Could you check a few things on this model? Use its own coordinates, in mm. Coordinates: 2 decimals unless noted, no trailing zeros. Loops run counter-clockwise (first coordinate to the right, second up) from the corner with the lowest first, then second, coordinate; pieces in that order, holes last. Notation, with made-up numbers: (-2, 22) -> (20, 22) arc R29 cw to (20, 55) -> close; hole circle Ø4 at (50.25, -5). An arc over 180 degrees is marked (long way). One line per question, with ' | ' between items.
Autodesk Inventor part; units mm, degrees
ref_plane "YZ Plane" through (0, 0, 0) normal (1, 0, 0) x (0, 1, 0)
ref_plane "XZ Plane" through (0, 0, 0) normal (0, 1, 0) x (-1, 0, 0)
ref_plane "XY Plane" through (0, 0, 0) normal (0, 0, 1) x (1, 0, 0)
sketch "Sketch2" plane through (0, 0, 0) normal (0, 0, 1) x (1, 0, 0)
  line L0 (0, 0) -> (200, 0)
  line L1 (200, 0) -> (200, 100)
  line L2 (200, 100) -> (0, 100)
  line L3 (0, 100) -> (0, 0)
  line L4 (0, 5) -> (200, 5) construction
  line L5 (0, 95) -> (200, 95) construction
  circle A0 centre (12.5, 95) radius 2.25
  circle A1 centre (12.5, 5) radius 2.25
  circle A2 centre (187.5, 95) radius 2.25
  circle A3 centre (187.5, 5) radius 2.25
  point P0 (23, 5)
  point P1 (23, 95)
  point P2 (53, 5)
  point P3 (53, 95)
  point P4 (85, 95)
  point P5 (85, 5)
  point P6 (115, 95)
  point P7 (115, 5)
  point P8 (147, 95)
  point P9 (147, 5)
  point P10 (177, 95)
  point P11 (177, 5)
  dimension "d18" = 90
  dimension "d0" = 200
  dimension "d1" = 100
  dimension "d2" = 30
  dimension "d3" = 32
  dimension "d4" = 30
  dimension "d5" = 32
  dimension "d6" = 30
  dimension "d13" = 10.5
  dimension "d15" = 10.5
  dimension "d16" = 12.5
  dimension "d17" = 175
  dimension "d21" = 4.5
  dimension "d22" = 4.5
  dimension "d23" = 4.5
  dimension "d24" = 4.5
extrude "Extrusion2" add sketch "Sketch2" along normal blind 20
hole "Hole1" at (23, 5, 0) at (23, 95, 0) at (53, 5, 0) at (53, 95, 0) at (85, 95, 0) at (85, 5, 0) at (115, 95, 0) at (115, 5, 0) at (147, 95, 0) at (147, 5, 0) at (177, 95, 0) at (177, 5, 0) direction (0, 0, 1) diameter 3.242 end through all
properties part number "3lasers1fiberHeatSinkBlock"
1) We'd pull the mould along Y, two halves only. Please class faces 1 (the face through (101, 100, 10)), 2 (the face through (189.58, 95.86, 9.86)), 3 (the face through (200, 49, 10)): pulls with the +Y half, pulls with the -Y half, needs draft (parallel to the pull), parting line crosses it, or undercut.
Data:
face 1: pulls with the +Y half | face 2: undercut | face 3: needs draft
2) If we section it at A-A on x = 187.5: Please give me the cut outline in (y, z).
Data:
outline: (0, 0) -> (2.75, 0) -> (2.75, 20) -> (0, 20) -> close; (7.25, 0) -> (92.75, 0) -> (92.75, 20) -> (7.25, 20) -> close; (97.25, 0) -> (100, 0) -> (100, 20) -> (97.25, 20) -> close
3) I need wall thicknesses on line 1 along Y through (x, z) = (85, 13.75); line 2 along Y through (x, z) = (187.5, 4.5). Which ranges of each line are inside material? Lowest first, please. Write a range as from..to.
Data:
line 1: 0..3.38, 6.62..93.38, 96.62..100 | line 2: 0..2.75, 7.25..92.75, 97.25..100
4) I'm going to push a flat-ended pin straight in: pin 1 Ø3 at (x, y) = (177, 95) entering from -Z. Where does the tip first touch, or does it pass through?
Data:
pin 1: through
